from build123d import *

# Parameters (mm, degrees)
BOSS_EXTRU_1_DEPTH           = 22.5
D_GAGEMENT_M51_D             = 5.5
D_GAGEMENT_M42_D             = 4.5
R_P_TITION_CIRCULAIRE2_COUNT = 4
CONG_1_R                     = 2
CHANFREIN1_SIZE              = 5
CONG_2_R                     = 4
ENL_V_MAT_EXTRU_1_REACH      = 92.057
ESQUISSE16_R                 = 13.5


with BuildPart() as part:
    # Esquisse1 → Boss.-Extru.1 (new, symmetric)
    with BuildSketch(Plane.XY):
        Polygon((52, 70), (50, 70), (50, 50), (0, 50), (0, 0), (50, 0), (50, -20), (52, -20), (52, 2), (2, 2), (2, 48), (52, 48), align=None)
    extrude(amount=BOSS_EXTRU_1_DEPTH, both=True)

    # Dégagement M51 (through all)
    with Locations(Plane.ZY.offset(-50)):
        with Locations((12.5, 60), (-12.5, 60), (-12.5, -10), (12.5, -10)):
            Hole(D_GAGEMENT_M51_D / 2)

    # Dégagement M42 (through all)
    with Locations(Plane.ZY):
        with Locations((0, 7)):
            d_gagement_m42 = Hole(D_GAGEMENT_M42_D / 2)

    # Répétition circulaire2: Dégagement M42 ×4 about axis
    r_p_tition_circulaire2_axis = Axis((0, 25, 0), (1, 0, 0))
    for i in range(1, R_P_TITION_CIRCULAIRE2_COUNT):
        add(d_gagement_m42.rotate(r_p_tition_circulaire2_axis, i * 360 / R_P_TITION_CIRCULAIRE2_COUNT), mode=Mode.SUBTRACT)

    # Congé1
    cong_1_edges = [part.edges().sort_by_distance(p)[0] for p in [
        (2, 48, 0),
        (2, 2, 0),
        (50, 0, 0),
        (50, 50, 0),
    ]]
    fillet(cong_1_edges, radius=CONG_1_R)

    # Chanfrein1
    chanfrein1_edges = [part.edges().sort_by_distance(p)[0] for p in [
        (51, -20, -22.5),
        (51, 70, -22.5),
        (51, -20, 22.5),
        (51, 70, 22.5),
    ]]
    chamfer(chanfrein1_edges, length=CHANFREIN1_SIZE)

    # Congé2
    cong_2_edges = [part.edges().sort_by_distance(p)[0] for p in [
        (52, 48, 0),
        (52, 2, 0),
        (0, 0, 0),
        (0, 50, 0),
    ]]
    fillet(cong_2_edges, radius=CONG_2_R)

    # Esquisse16 → Enlèv. mat.-Extru.1 (cut, up to next)
    with BuildSketch(Plane.ZY, mode=Mode.PRIVATE) as enl_v_mat_extru_1_sk1:
        with Locations(Location((0, 25, 0), (0, 0, 270))):
            Circle(ESQUISSE16_R)
    enl_v_mat_extru_1_tool1 = extrude(enl_v_mat_extru_1_sk1.sketch, amount=-ENL_V_MAT_EXTRU_1_REACH, mode=Mode.PRIVATE) & part.part
    add(enl_v_mat_extru_1_tool1.solids().sort_by_distance((0, 25, 0))[0], mode=Mode.SUBTRACT)


solid = part.part
Geometry check sheet. Reference: the model listing, model coordinates, mm. A direction names the side the tool comes from. Give positions to 0.01 mm unless a question says otherwise; leave off trailing zeros. Write each loop counter-clockwise with the first axis right and the second up, starting at its lowest first coordinate (ties: lowest second). Pieces come first, ordered by that corner, then holes. Notation, with made-up numbers: (55.25, -1) - (62.25, -1) arc R36 cw to (62.25, 38) - close; hole circle Ø4 at (33, -22). An arc over 180 degrees is marked (long way). Put each result on its own line as item: value.
1. Sectioned sample at A-A, the plane x = 46.5. Enter the section's corners in (y, z).
Ans:
outline: (0, -22.5) - (2, -22.5) - (2, 22.5) - (0, 22.5) - close; (48, -22.5) - (50, -22.5) - (50, 22.5) - (48, 22.5) - close
2. Sectioned sample at C-C, the plane y = 43. Enter the section's corners in (x, z), plus the area to 3 significant figures.
Ans:
outline: (0, -22.5) - (2, -22.5) - (2, -2.25) - (0, -2.25) - close; (0, 2.25) - (2, 2.25) - (2, 22.5) - (0, 22.5) - close
area: 81.0 mm²
3. Sectioned sample at D-D, the plane z = 19. Enter the section's corners in (x, y), plus the area to 3 significant figures.
Ans:
outline: (0, 4) arc R4 ccw to (4, 0) - (48, 0) arc R2 cw to (50, -2) - (50, -18.5) - (52, -18.5) - (52, -2) arc R4 ccw to (48, 2) - (4, 2) arc R2 cw to (2, 4) - (2, 22.98) - (0, 22.98) - close; (0, 27.02) - (2, 27.02) - (2, 46) arc R2 cw to (4, 48) - (48, 48) arc R4 ccw to (52, 52) - (52, 68.5) - (50, 68.5) - (50, 52) arc R2 cw to (48, 50) - (4, 50) arc R4 ccw to (0, 46) - close
area: 356 mm²
4. Thickness scan on line 1 (Y direction, x = 18.5, z = -5); line 2 (Y direction, x = 51, z = -12); line 3 (Z direction, x = 0.9, y = 43). Record the ranges inside material, lowest first.
Ans:
line 1: y = 0 to 2, 48 to 50
line 2: y = -20 to -12.7, -7.3 to 0.65, 49.35 to 57.3, 62.7 to 70
line 3: z = -22.5 to -2.25, 2.25 to 22.5
5. Go/stop test with flat-tipped pins: pin 1 (1.5 mm diameter, centred on x = 17.5, z = 12.5, fed in from +Y); pin 2 (14.5 mm diameter, centred on y = -10, z = 9.5, fed in from -X); pin 3 (4 mm diameter, centred on y = 38, z = 4.5, fed in from +X). Record where each tip stops, or that it passes through.
Ans:
pin 1: stops at y = 50
pin 2: stops at x = 50
pin 3: stops at x = 2
6. Draft check along Y on faces 1 (the flat face through (51, 70, 0)), 2 (the flat face through (1, 25, 22.5)), 3 (the cylindrical face through (49.4, -0.57, 0.32)), 4 (the cylindrical face through (2.6, 2.57, 0.32)). Enter one of: +Y half, -Y half, draft (parallel to the pull), parting line (faces both ways), or undercut.
Ans:
face 1: +Y half
face 2: draft
face 3: -Y half
face 4: undercut
7. Set-up check for faces 5 (the cylindrical face through (2.57, 47.4, -0.32)), 6 (the cylindrical face through (1.203, 48.859, 0.315)): record each of +Z, -Z, +X, -X, +Y, -Y from which the full face is reachable in a straight line by a thin tool's end or side.
Ans:
face 5: +Z, -Z, +X
face 6: +Z, -Z, -X, +Y
8. Sectioned sample at B-B, the plane y = 60. Enter the section's corners in (x, z).
Ans:
outline: (50, -22.5) - (52, -22.5) - (52, -15.25) - (50, -15.25) - close; (50, -9.75) - (52, -9.75) - (52, 9.75) - (50, 9.75) - close; (50, 15.25) - (52, 15.25) - (52, 22.5) - (50, 22.5) - close
